from build123d import *

# Parameters (mm, degrees)
F0_R     = 3.9751
F1_DEPTH = 2.7178
F2_W     = 5.207
F2_H     = 2.6416
F3_DEPTH = 2.7432


with BuildPart() as f1:
    # F0 (on Top) → F1 (new body)
    with BuildSketch(Plane.XY):
        with BuildLine():
            Line((8.4201, 9.4996), (-8.4201, 9.4996))
            ThreePointArc((-8.4201, 9.4996), (-10.216151, 8.755651), (-10.9601, 6.9596))
            Line((-10.9601, 6.9596), (-10.9601, -6.9596))
            ThreePointArc((-10.9601, -6.9596), (-10.216151, -8.755651), (-8.4201, -9.4996))
            Line((-8.4201, -9.4996), (8.4201, -9.4996))
            ThreePointArc((8.4201, -9.4996), (10.216151, -8.755651), (10.9601, -6.9596))
            Line((10.9601, -6.9596), (10.9601, 6.9596))
            ThreePointArc((10.9601, 6.9596), (10.216151, 8.755651), (8.4201, 9.4996))
        make_face()
        with Locations((1.9558, 0)):
            Circle(F0_R, mode=Mode.SUBTRACT)
    extrude(amount=F1_DEPTH)

    # F2 (on face) → F3 (join)
    with BuildSketch(Plane.XY.offset(2.7178)):
        with BuildLine():
            Line((0.8255, 9.4996), (-6.5151, 9.4996))
            Line((-6.5151, 9.4996), (-6.5151, 8.128))
            ThreePointArc((-6.5151, 8.128), (-6.143126, 7.229974), (-5.2451, 6.858))
            Line((-5.2451, 6.858), (0.8255, 6.858))
            Line((0.8255, 6.858), (0.8255, 9.4996))
        make_face()
        with BuildLine():
            Line((8.2677, 9.4996), (3.0607, 9.4996))
            Line((3.0607, 9.4996), (3.0607, 6.858))
            Line((3.0607, 6.858), (6.9977, 6.858))
            ThreePointArc((6.9977, 6.858), (7.895726, 7.229974), (8.2677, 8.128))
            Line((8.2677, 8.128), (8.2677, 9.4996))
        make_face()
        with BuildLine():
            Line((-6.5151, -8.128), (-6.5151, -9.4996))
            Line((-6.5151, -9.4996), (0.8382, -9.4996))
            Line((0.8382, -9.4996), (0.8382, -6.858))
            Line((0.8382, -6.858), (-5.2451, -6.858))
            ThreePointArc((-5.2451, -6.858), (-6.143126, -7.229974), (-6.5151, -8.128))
        make_face()
        with Locations((5.6642, -8.1788)):
            Rectangle(F2_W, F2_H)
    extrude(amount=F3_DEPTH)


solid = f1.part
Design review of the part built by this model. Coordinates are the model's own, in mm. A direction names the side the tool comes from. Give positions to 0.01 mm unless a question says otherwise; leave off trailing zeros. Loops run counter-clockwise (first coordinate to the right, second up) from the corner with the lowest first, then second, coordinate; pieces in that order, holes last. Notation, with made-up numbers: (57.5, 19) - (78.5, 19) arc R21 cw to (78.5, 36) - close; hole circle Ø7 at (27, -24). An arc over 180 degrees is marked (long way). Write item = value, one per line.
1) Take a section at C-C on x = -4.5. State the section outline as (y, z) points, and give its area (3 significant figures).
Result sheet:
outline = (-9.5, 0) - (9.5, 0) - (9.5, 5.46) - (6.86, 5.46) - (6.86, 2.72) - (-6.86, 2.72) - (-6.86, 5.46) - (-9.5, 5.46) - close
area = 66.1 mm2
2) To check wall thickness, follow line 1 (Y direction, x = -1.25, z = 3.25); line 2 (Z direction, x = -0.75, y = -4.5); line 3 (Y direction, x = -1.5, z = 1.6). State the ranges of each line that lie inside material, in increasing order.
Result sheet:
line_1 = -9.5 to -6.86, 6.86 to 9.5
line_2 = 0 to 2.72
line_3 = -9.5 to -1.96, 1.96 to 9.5
3) Take a section at D-D on z = 0.7. State the section outline as (x, y) points.
Result sheet:
outline = (-10.96, -6.96) arc R2.54 ccw to (-8.42, -9.5) - (8.42, -9.5) arc R2.54 ccw to (10.96, -6.96) - (10.96, 6.96) arc R2.54 ccw to (8.42, 9.5) - (-8.42, 9.5) arc R2.54 ccw to (-10.96, 6.96) - close; hole circle Ø7.95 at (1.96, 0)
4) Take a section at B-B on y = 0. State the section outline as (x, z) points.
Result sheet:
outline = (-10.96, 0) - (-2.02, 0) - (-2.02, 2.72) - (-10.96, 2.72) - close; (5.93, 0) - (10.96, 0) - (10.96, 2.72) - (5.93, 2.72) - close
5) Take a section at A-A on z = 4.1. State the section outline as (x, y) points, and give its area (3 significant figures).
Result sheet:
outline = (-6.52, -9.5) - (0.84, -9.5) - (0.84, -6.86) - (-5.25, -6.86) arc R1.27 ccw to (-6.52, -8.13) - close; (-6.52, 8.13) arc R1.27 ccw to (-5.25, 6.86) - (0.83, 6.86) - (0.83, 9.5) - (-6.52, 9.5) - close; (3.06, -9.5) - (8.27, -9.5) - (8.27, -6.86) - (3.06, -6.86) - close; (3.06, 6.86) - (7, 6.86) arc R1.27 ccw to (8.27, 8.13) - (8.27, 9.5) - (3.06, 9.5) - close
area = 65.3 mm2
6) Draft analysis for pull direction Y (two halves, no side actions). For faces 1 (the face through (-10.196, 8.775, 1.34)), 2 (the face through (5.63, -1.52, 1.34)), 3 (the face through (6, -6.858, 4)), 4 (the face through (6, 8, 5.461)), state which applies: +Y half, -Y half, draft (parallel to the pull), parting line (faces both ways), or undercut.
Result sheet:
face_1 = +Y half
face_2 = undercut
face_3 = undercut
face_4 = draft
7) Clearance check with flat-ended pins moving along their axes: pin 1 Ø5.5 at (x, y) = (-2.5, 1.5) entering from +Z; pin 2 Ø1 at (y, z) = (2, 4.5) entering from -X; pin 3 Ø1.3 at (y, z) = (8.5, 4.5) entering from +X; pin 4 Ø1.3 at (y, z) = (-8.5, 4.5) entering from -X. State where each tip first meets the part, or that it passes through.
Result sheet:
pin_1 = 2.72
pin_2 = through
pin_3 = 8.27
pin_4 = -6.52
8) Tool access review of faces 5 (the face through (5, 6.858, 4)), 6 (the face through (3.061, 8, 4)), 7 (the face through (8.268, 9, 4)): name each direction out of +Z, -Z, +X, -X, +Y, -Y from which nothing blocks a thin tool from reaching the whole face with its end or side.
Result sheet:
face_5 = +Z, +X, -X
face_6 = +Z, +Y, -Y
face_7 = +Z, +X, +Y, -Y
